```python
from build123d import *

# Parameters (mm, degrees)
SKIZZE1_W                       = 100
SKIZZE1_H                       = 100
AUFSATZ_LINEAR_AUSTRAGEN1_DEPTH = 200
WANDUNG1_T                      = -3
FASE1_SIZE                      = 150
FASE1_SIZE2                     = 86.602540378
FASE1_PART_2_SIZE               = 150
FASE1_PART_2_SIZE2              = 86.602540378
BOHRUNG1_D                      = 25.4
BOHRUNG1_DEPTH                  = 3
BOHRUNG1_ON_FACE_2_D            = 25.4
BOHRUNG1_ON_FACE_2_DEPTH        = 3
DURCHGANGSLOCH_F_R_M101_D       = 11
DURCHGANGSLOCH_F_R_M101_DEPTH   = 3


with BuildPart() as part:
    # Skizze1 → Aufsatz-Linear austragen1 (new body)
    with BuildSketch(Plane(origin=(0, 0, 0), x_dir=(1, 0, 0), z_dir=(0, 1, 0))):
        with Locations((50, 50)):
            Rectangle(SKIZZE1_W, SKIZZE1_H)
    extrude(amount=AUFSATZ_LINEAR_AUSTRAGEN1_DEPTH)

    # Wandung1
    wandung1_openings = [part.faces().sort_by_distance(p)[0] for p in [
        (50, 200, -50),
        (50, 100, -100),
        (0, 100, -50),
    ]]
    offset(amount=WANDUNG1_T, openings=wandung1_openings, kind=Kind.INTERSECTION)

    # Fase1
    fase1_edges = [part.edges().sort_by_distance(p)[0] for p in [
        (98.5, 200, -100),
    ]]
    fase1_side = [part.faces().sort_by_distance(p)[0] for p in [
        (98.5, 197.763932023, -100),
    ]]
    chamfer(fase1_edges, length=FASE1_SIZE, length2=FASE1_SIZE2, reference=fase1_side[0])

    # Fase1 part 2
    fase1_part_2_edges = [part.edges().sort_by_distance(p)[0] for p in [
        (0, 200, -1.5),
    ]]
    fase1_part_2_side = [part.faces().sort_by_distance(p)[0] for p in [
        (0, 1.5, -97.763932023),
    ]]
    chamfer(fase1_part_2_edges, length=FASE1_PART_2_SIZE, length2=FASE1_PART_2_SIZE2, reference=fase1_part_2_side[0])

    # Bohrung1
    with Locations(Plane(origin=(100, 70, -40), x_dir=(0, 0, 1), z_dir=(1, 0, 0))):
        with Locations((0, 0)):
            Hole(BOHRUNG1_D / 2, depth=BOHRUNG1_DEPTH)

    # Bohrung1 on face 2
    with Locations(Plane(origin=(60, 70, 0), x_dir=(1, 0, 0), z_dir=(0, 0, 1))):
        with Locations((0, 0)):
            Hole(BOHRUNG1_ON_FACE_2_D / 2, depth=BOHRUNG1_ON_FACE_2_DEPTH)

    # Durchgangsloch für M101
    with Locations(Plane(origin=(0, 0, 0), x_dir=(-1, 0, 0), z_dir=(0, -1, 0))):
        with Locations((-90, 90), (-90, 10), (-60, 10), (-10, 10)):
            Hole(DURCHGANGSLOCH_F_R_M101_D / 2, depth=DURCHGANGSLOCH_F_R_M101_DEPTH)


solid = part.part
```
Verification items for the finished model (mm, model axes). A direction names the side the tool comes from. Coordinates: 2 decimals unless noted, no trailing zeros. Loops run counter-clockwise (first coordinate to the right, second up) from the corner with the lowest first, then second, coordinate; pieces in that order, holes last. Notation, with made-up numbers: (-19.5, 28) - (17.5, 28) arc R30 ccw to (17.5, 51) - close; hole circle Ø6 at (36, -15.5). An arc over 180 degrees is marked (long way). Answer as a JSON object with one key per item and string values.
(1) Access from +Z, -Z, +X, -X, +Y, -Y to the whole of each face (thin tool, end or side, straight path). Record for faces 5 (the cylindrical face through (54.505, 1.521, -10.242)), 6 (the flat face through (48, 3, -52)).
Response:
{"face 5": "+Y, -Y", "face 6": "-Z, -X, +Y"}
(2) Cross-section at B-B, the plane y = 70. Record the boundary of the cut face in (x, z).
Response:
{"outline": "(11.55, -3) - (47.3, -3) - (47.3, 0) - (11.55, 0) - close; (72.7, -3) - (97, -3) - (97, -27.3) - (100, -27.3) - (100, 0) - (72.7, 0) - close; (97, -88.45) - (100, -88.45) - (100, -52.7) - (97, -52.7) - close"}
(3) Cross-section at C-C, the plane x = 90. Record the boundary of the cut face in (y, z).
Response:
{"outline": "(0, -100) - (3, -100) - (3, -95.5) - (0, -95.5) - close; (0, -84.5) - (3, -84.5) - (3, -15.5) - (0, -15.5) - close; (0, -4.5) - (3, -4.5) - (3, -3) - (200, -3) - (200, 0) - (0, 0) - close"}
(4) Cross-section at A-A, the plane z = -10. Record the boundary of the cut face in (x, y).
Response:
{"outline": "(0, 0) - (4.5, 0) - (4.5, 3) - (0, 3) - close; (15.5, 0) - (54.5, 0) - (54.5, 3) - (15.5, 3) - close; (65.5, 0) - (84.5, 0) - (84.5, 3) - (65.5, 3) - close; (95.5, 0) - (100, 0) - (100, 200) - (97, 200) - (97, 3) - (95.5, 3) - close"}
(5) Mould release check, pull along Y, two halves, no side actions. Record for faces 1 (the cylindrical face through (47.886, 73.815, -1.521)), 2 (the flat face through (43.907, 126.05, -1.479)), 3 (the flat face through (100, 76, -27)), 4 (the cylindrical face through (98.479, 66.185, -52.114)): pulls with the +Y half, pulls with the -Y half, needs draft (parallel to the pull), parting line crosses it, or undercut.
Response:
{"face 1": "undercut", "face 2": "pulls with the +Y half", "face 3": "needs draft", "face 4": "undercut"}
(6) Scan lines: line 1 along Z through (x, y) = (90, 1); line 2 along X through (y, z) = (74, -70.5); line 3 along Y through (x, z) = (19.5, -68). Record each from-to range of solid material in increasing order.
Response:
{"line 1": "z = -100 to -95.5, -84.5 to -15.5, -4.5 to 0", "line 2": "x = 97 to 100", "line 3": "y = 0 to 3"}
(7) Go/stop test with flat-tipped pins: pin 1 Ø9 at (x, z) = (90, -10) entering from +Y; pin 2 Ø2 at (x, y) = (19.5, 25.5) entering from -Z; pin 3 Ø1.5 at (y, z) = (23, -16) entering from -X. Record where each tip stops, or that it passes through.
Response:
{"pin 1": "passes through", "pin 2": "stops at z = -3", "pin 3": "stops at x = 97"}
(8) Cross-section at D-D, the plane x = 68. Record the boundary of the cut face in (y, z).
Response:
{"outline": "(0, -100) - (3, -100) - (3, -3) - (60.14, -3) - (60.14, 0) - (0, 0) - close; (79.86, -3) - (167.78, -3) - (167.78, 0) - (79.86, 0) - close"}
